Geometry check sheet. Reference: drawing and pictorial views, mm from the part's lowest x, y, z. Give positions to 0.01 mm unless a question says otherwise; leave off trailing zeros. Order: outer loops, then holes, each group sorted by start corner. A loop starts at its lowest first (then second) coordinate and runs counter-clockwise, first axis right, second up. Notation, with made-up numbers: (-36.75, -12) - (-3.75, -12) arc R30 cw to (-3.75, 11) - close; hole circle Ø2 at (68, -2.5). An arc over 180 degrees is marked (long way). Answer as a JSON object with one key per item and string values.
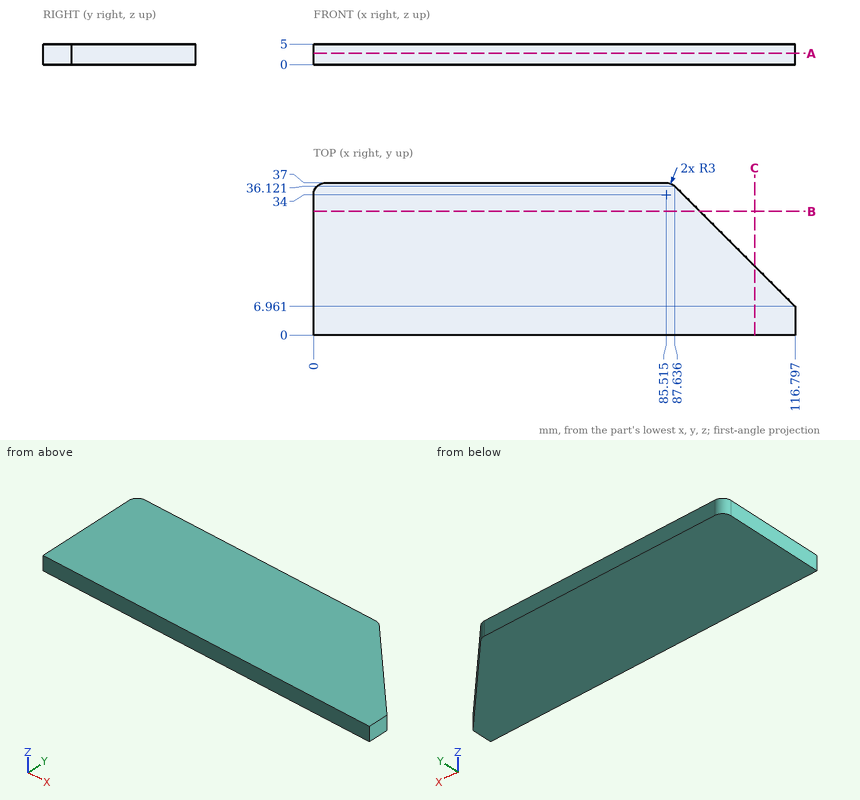
(1) Material ranges on line 1 along X through (y, z) = (31.5, 1); line 2 along X through (y, z) = (7, 4.4); line 3 along Y through (x, z) = (93.5, 2.6), recorded low to high. Write a range as [from, to].
Computed values:
{"line 1": "x = [0, 92.26]", "line 2": "x = [0, 116.76]", "line 3": "y = [0, 30.26]"}
(2) Gauge pin test, flat end, axial feed: pin 1 Ø8 at (x, y) = (99, 15.5) entering from -Z. Record the tip position at first contact, or that the pin passes through.
Computed values:
{"pin 1": "stops at z = 0"}
(3) Section check A-A (z = 2.7). Record the cut outline in (x, y) (1 decimal).
Computed values:
{"outline": "(0, 0) - (116.8, 0) - (116.8, 7) - (87.6, 36.1) arc R3 ccw to (85.5, 37) - (3, 37) arc R3 ccw to (0, 34) - close"}
(4) Section check B-B (y = 30). Record the cut outline in (x, z).
Computed values:
{"outline": "(0, 0) - (93.76, 0) - (93.76, 5) - (0, 5) - close"}
(5) Section check C-C (x = 107). Record the cut outline in (y, z), then the cut area to 3 significant figures.
Computed values:
{"outline": "(0, 0) - (16.76, 0) - (16.76, 5) - (0, 5) - close", "area": "83.8 mm²"}
